Autodesk Inventor part; units mm, degrees
ref_plane "YZ Plane" through (0, 0, 0) normal (1, 0, 0) x (0, 1, 0)
ref_plane "XZ Plane" through (0, 0, 0) normal (0, 1, 0) x (-1, 0, 0)
ref_plane "XY Plane" through (0, 0, 0) normal (0, 0, 1) x (1, 0, 0)
sketch "Sketch1" plane through (0, 0, 0) normal (0, 0, 1) x (1, 0, 0)
  line L0 (-40, -40) -> (40, -40)
  line L1 (40, -40) -> (40, 40)
  line L2 (40, 40) -> (-40, 40)
  line L3 (-40, 40) -> (-40, -40)
  line L4 (-40, -40) -> (40, 40) construction
  line L5 (40, -40) -> (-40, 40) construction
  line L6 (-2.8, -18.3) -> (2.8, -18.3)
  line L7 (2.8, -18.3) -> (2.8, 18.3)
  line L8 (2.8, 18.3) -> (-2.8, 18.3)
  line L9 (-2.8, 18.3) -> (-2.8, -18.3)
  line L10 (-2.8, -18.3) -> (2.8, 18.3) construction
  line L11 (2.8, -18.3) -> (-2.8, 18.3) construction
  circle A0 centre (23, 6) radius 1.8
  line L12 (0, 56) -> (0, -56) construction
  circle A1 centre (-23, 6) radius 1.8
  point P0 (0, 0)
  dimension "d0" = 80
  dimension "d1" = 80
  dimension "d2" = 5.6
  dimension "d3" = 36.6
  dimension "d4" = 3.6
  dimension "d5" = 12.3
  dimension "d6" = 23
extrude "Extrusion1" add sketch "Sketch1" along normal blind 3
fillet "Fillet1" radius 13.5 4 edges at (40, 40, 1.5) (40, -40, 1.5) (-40, -40, 1.5) (-40, 40, 1.5)
chamfer "Chamfer1" distance 1.7 angle 45 2 edges at (-24.8, 6, 3) (21.2, 6, 3)
chamfer "Chamfer2" distance 0.3 angle 45 25 edges at (-40, 0, 0) (-36.0459, -36.0459, 0) (0, -40, 0) (36.0459, -36.0459, 0) (40, 0, 0) (36.0459, 36.0459, 0) (0, 40, 0) (-36.0459, 36.0459, 0) (-40, 0, 3) (-36.0459, -36.0459, 3) (0, -40, 3) (36.0459, -36.0459, 3) (40, 0, 3) (36.0459, 36.0459, 3) (0, 40, 3) (-36.0459, 36.0459, 3) (-2.8, 0, 3) (2.8, 0, 3) (0, 18.3, 3) (2.8, 0, 0) (0, -18.3, 3) (0, 18.3, 0) (0, -18.3, 0) (-24.8, 6, 0) (21.2, 6, 0)
properties part number "TopV3Back"
For this review, take the finished solid that the model builds, in its own axes (mm). A direction names the side the tool comes from. Round coordinates to 2 decimals unless told otherwise and drop trailing zeros. Loops run counter-clockwise (first coordinate to the right, second up) from the corner with the lowest first, then second, coordinate; pieces in that order, holes last.
Q1. Insertion check: pin 1 Ø3 at (x, y) = (23, 6) entering from -Z. The pin has a flat end and moves straight along its axis. Give the tip position at first contact, or say it passes through.
Result sheet:
pin 1: passes through
Q2. To check wall thickness, follow line 1 along Y through (x, z) = (-2, 0.35); line 2 along X through (y, z) = (-9, 1.9); line 3 along Y through (x, z) = (23, 0.9). State the ranges of each line that lie inside material, in increasing order.
Result sheet:
line 1: y = -40 to -18.3, 18.3 to 40
line 2: x = -40 to -2.8, 2.8 to 40
line 3: y = -40 to 4.2, 7.8 to 40
Q3. Mouldability with a two-part tool opening along X and no side actions: class faces 1 (the face through (24.663, 6.689, 0.793)), 2 (the face through (-40, 0, 1)), 3 (the face through (35.814, 36.021, 2.881)), 4 (the face through (21.487, 4.84, 1.406)) as +X half, -X half, draft (parallel to the pull), parting line (faces both ways), or undercut.
Result sheet:
face 1: undercut
face 2: -X half
face 3: +X half
face 4: undercut
Q4. Add section B-B on x = 23. Write out the cut boundary in (y, z).
Result sheet:
outline: (-40, 0.3) - (-39.7, 0) - (3.9, 0) - (4.2, 0.3) - (4.2, 1.3) - (2.5, 3) - (-39.7, 3) - (-40, 2.7) - close; (7.8, 0.3) - (8.1, 0) - (39.7, 0) - (40, 0.3) - (40, 2.7) - (39.7, 3) - (9.5, 3) - (7.8, 1.3) - close
Q5. Add section A-A on y = 16.5. Write out the cut boundary in (x, z).
Result sheet:
outline: (-40, 0.3) - (-39.7, 0) - (-2.8, 0) - (-2.8, 2.7) - (-3.1, 3) - (-39.7, 3) - (-40, 2.7) - close; (2.8, 0.3) - (3.1, 0) - (39.7, 0) - (40, 0.3) - (40, 2.7) - (39.7, 3) - (3.1, 3) - (2.8, 2.7) - close
Q6. Add section C-C on y = 6. Give the number of separate pieces and of enclosed holes in the cut face, plus the area to 3 significant figures.
Result sheet:
separate pieces: 4
enclosed holes: 0
area: 195 mm2
Q7. Machinability: for faces 5 (the face through (-35.814, -36.021, 2.881)), 6 (the face through (0, 18.3, 1)), which of the approach directions +Z, -Z, +X, -X, +Y, -Y give a long, thin tool a straight path to every point of the face, cutting with its end or side? Answer none if there is none.
Result sheet:
face 5: +Z, -X, -Y
face 6: +Z, -Z
